```python
from build123d import *

# Parameters (mm, degrees)
SKETCH1_R           = 1.75
BOSS_EXTRUDE1_DEPTH = 2


with BuildPart() as part:
    # Sketch1 → Boss-Extrude1 (new body)
    with BuildSketch(Plane(origin=(0, 0, 0), x_dir=(1, 0, 0), z_dir=(0, 1, 0))):
        Polygon((-37.5, 16.15), (25.5, 16.15), (25.5, 52.15), (40.5, 52.15), (40.5, -52.15), (25.5, -52.15), (25.5, -16.15), (-37.5, -16.15), (-37.5, -2), (-20.5, -2), (-20.5, -10.5), (20.5, -10.5), (20.5, 10.5), (-20.5, 10.5), (-20.5, 2), (-37.5, 2), align=None)
        with Locations((-24.5, 4.8)):
            Circle(SKETCH1_R, mode=Mode.SUBTRACT)
        with Locations((-24.5, -4.8)):
            Circle(SKETCH1_R, mode=Mode.SUBTRACT)
        with Locations((24.5, -4.8)):
            Circle(SKETCH1_R, mode=Mode.SUBTRACT)
        with Locations((24.5, 4.8)):
            Circle(SKETCH1_R, mode=Mode.SUBTRACT)
    extrude(amount=BOSS_EXTRUDE1_DEPTH)


solid = part.part
```
Geometry check sheet. Reference: the model listing, model coordinates, mm. A direction names the side the tool comes from. Round coordinates to 2 decimals unless told otherwise and drop trailing zeros. Loops run counter-clockwise (first coordinate to the right, second up) from the corner with the lowest first, then second, coordinate; pieces in that order, holes last. Notation, with made-up numbers: (68.25, -30) - (110.25, -30) arc R31 ccw to (110.25, 0) - close; hole circle Ø2 at (-15, -22). An arc over 180 degrees is marked (long way). Write each question's results on one line, items separated by ' | '. Start each with the question number.
Q1. Release check for a two-part mould opening along X. For faces 4 (the flat face through (25.5, 1, -34)), 5 (the flat face through (40.5, 1, -1)), 6 (the flat face through (-6, 1, 16.15)), 7 (the flat face through (0, 1, -10.5)) record: +X half, -X half, draft (parallel to the pull), parting line (faces both ways), or undercut.
Q2. Cross-section at B-B on y = 0.55. Enter the section's corners in (x, z), and give its area (3 significant figures).
Q3. Cross-section at A-A on x = 19. Enter the section's corners in (y, z), and give its area (3 significant figures).
Q4. Access from +Z, -Z, +X, -X, +Y, -Y to the whole of each face (thin tool, end or side, straight path). Record for faces 1 (the flat face through (-29, 1, 2)), 2 (the flat face through (-20.5, 1, -6)), 3 (the flat face through (-6, 1, -16.15)).
Q5. Cross-section at C-C on z = 8. Enter the section's corners in (x, y).
Q6. Cross-section at D-D on z = -4.8. Enter the section's corners in (x, y).
Q7. Gauge pin test, flat ends, axial feed: P1, Ø1, axis at x = -8, y = 1, coming from the -Z side; P2, Ø3, axis at x = 24.5, z = 4.8, coming from the +Y side; P3, Ø1, axis at y = 1, z = -38.5, coming from the -X side; P4, Ø1, axis at x = -3, y = 0.5, coming from the +Z side. Record the tip position at first contact, or that the pin passes through.
Q8. Thickness scan on line 1 (Z direction, x = -24.5, y = 1); line 2 (X direction, y = 0.75, z = 4.8); line 3 (Z direction, x = 24.5, y = 0.55). Record the ranges inside material, lowest first. Write a range as [from, to].
Answers below:
1) face 4: -X half | face 5: +X half | face 6: draft | face 7: undercut
2) outline: (-37.5, -16.15) - (25.5, -16.15) - (25.5, -52.15) - (40.5, -52.15) - (40.5, 52.15) - (25.5, 52.15) - (25.5, 16.15) - (-37.5, 16.15) - (-37.5, 2) - (-20.5, 2) - (-20.5, 10.5) - (20.5, 10.5) - (20.5, -10.5) - (-20.5, -10.5) - (-20.5, -2) - (-37.5, -2) - close; hole circle Ø3.5 at (-24.5, -4.8); hole circle Ø3.5 at (-24.5, 4.8); hole circle Ø3.5 at (24.5, -4.8); hole circle Ø3.5 at (24.5, 4.8) | area: 2,630 mm²
3) outline: (0, -16.15) - (2, -16.15) - (2, -10.5) - (0, -10.5) - close; (0, 10.5) - (2, 10.5) - (2, 16.15) - (0, 16.15) - close | area: 22.6 mm²
4) face 1: -X, +Y, -Y | face 2: +Y, -Y | face 3: -Z, -X, +Y, -Y
5) outline: (-37.5, 0) - (-20.5, 0) - (-20.5, 2) - (-37.5, 2) - close; (20.5, 0) - (40.5, 0) - (40.5, 2) - (20.5, 2) - close
6) outline: (-37.5, 0) - (-26.25, 0) - (-26.25, 2) - (-37.5, 2) - close; (-22.75, 0) - (-20.5, 0) - (-20.5, 2) - (-22.75, 2) - close; (20.5, 0) - (22.75, 0) - (22.75, 2) - (20.5, 2) - close; (26.25, 0) - (40.5, 0) - (40.5, 2) - (26.25, 2) - close
7) P1: stops at z = -16.15 | P2: passes through | P3: stops at x = 25.5 | P4: stops at z = 16.15
8) line 1: z = [-16.15, -6.55], [-3.05, -2], [2, 3.05], [6.55, 16.15] | line 2: x = [-37.5, -26.25], [-22.75, -20.5], [20.5, 22.75], [26.25, 40.5] | line 3: z = [-16.15, -6.55], [-3.05, 3.05], [6.55, 16.15]
